```python
from build123d import *

# Parameters (mm, degrees)
SKETCH1_R           = 49.685
BOSS_EXTRUDE1_DEPTH = 5
SKETCH2_R           = 46.685
CUT_EXTRUDE1_DEPTH  = 3
SKETCH3_W           = 7
SKETCH3_H           = 5
SKETCH3_W_2         = 5
SKETCH3_H_2         = 7
BOSS_EXTRUDE2_DEPTH = 2
SKETCH4_R           = 40
BOSS_EXTRUDE3_DEPTH = 54.61
FILLET2_R           = 3
FILLET3_R           = 40


with BuildPart() as part:
    # Sketch1 → Boss-Extrude1 (new body)
    with BuildSketch(Plane.XY):
        Circle(SKETCH1_R)
    extrude(amount=BOSS_EXTRUDE1_DEPTH)

    # Sketch2 → Cut-Extrude1 (cut)
    with BuildSketch(Plane.XY.offset(5)):
        Circle(SKETCH2_R)
    extrude(amount=-CUT_EXTRUDE1_DEPTH, mode=Mode.SUBTRACT)

    # Sketch3 → Boss-Extrude2 (add)
    with BuildSketch(Plane(origin=(0, 0, 0), x_dir=(-1, 0, 0), z_dir=(0, 0, -1))):
        Polygon((-37.72768231, 37.72768231), (-67.675, 0), (-37.72768231, -37.72768231), (0, -67.675), (37.72768231, -37.72768231), (67.675, 0), (37.72768231, 37.72768231), (0, 67.675), align=None)
        with Locations((-57.675, 0)):
            Rectangle(SKETCH3_W, SKETCH3_H, mode=Mode.SUBTRACT)
        with Locations((0, 57.675)):
            Rectangle(SKETCH3_W_2, SKETCH3_H_2, mode=Mode.SUBTRACT)
        with Locations((57.675, 0)):
            Rectangle(SKETCH3_W, SKETCH3_H, mode=Mode.SUBTRACT)
        with Locations((0, -57.675)):
            Rectangle(SKETCH3_W_2, SKETCH3_H_2, mode=Mode.SUBTRACT)
    extrude(amount=BOSS_EXTRUDE2_DEPTH)

    # Sketch4 → Boss-Extrude3 (add)
    with BuildSketch(Plane(origin=(0, 0, -2), x_dir=(-1, 0, 0), z_dir=(0, 0, -1))):
        Circle(SKETCH4_R)
    extrude(amount=BOSS_EXTRUDE3_DEPTH)

    # Fillet2
    fillet2_edges = [part.edges().sort_by_distance(p)[0] for p in [
        (-67.675, 0, -1),
        (0, 67.675, -1),
        (67.675, 0, -1),
        (0, -67.675, -1),
    ]]
    fillet(fillet2_edges, radius=FILLET2_R)

    # Fillet3
    fillet3_edges = [part.edges().sort_by_distance(p)[0] for p in [
        (-37.72768231, 37.72768231, -1),
        (37.72768231, 37.72768231, -1),
        (37.72768231, -37.72768231, -1),
        (-37.72768231, -37.72768231, -1),
    ]]
    fillet(fillet3_edges, radius=FILLET3_R)


solid = part.part
```
Geometry check sheet. Reference: the model listing, model coordinates, mm. A direction names the side the tool comes from. Give positions to 0.01 mm unless a question says otherwise; leave off trailing zeros. Write each loop counter-clockwise with the first axis right and the second up, starting at its lowest first coordinate (ties: lowest second). Pieces come first, ordered by that corner, then holes. Notation, with made-up numbers: (72, 84.5) - (101, 84.5) arc R11 cw to (101, 90.5) - close; hole circle Ø5 at (84.25, 11.5). An arc over 180 degrees is marked (long way). Use a Markdown table: item, result.
Q1. Thickness scan on L1, parallel to Y at x = 0, z = 3.8 (3 decimals); L2, parallel to Z at x = -6, y = -7.5; L3, parallel to Z at x = -24.5, y = 44. Record the ranges inside material, lowest first. Write a range as [from, to].
Computed:
| item | result |
|---|---|
| L1 | y = [-49.685, -46.685], [46.685, 49.685] |
| L2 | z = [-56.61, 2] |
| L3 | z = [-2, 0] |
Q2. Go/stop test with flat-tipped pins: P1, Ø10, axis at y = 46, z = -12.5, coming from the -X side; P2, Ø2, axis at y = 26.5, z = -32.5, coming from the -X side; P3, Ø1.6, axis at x = 1, z = -0.5, coming from the -Y side; P4, Ø1, axis at y = -57.5, z = -1, coming from the -X side. Record where each tip stops, or that it passes through.
Computed:
| item | result |
|---|---|
| P1 | passes through |
| P2 | stops at x = -30.82 |
| P3 | stops at y = -66.84 |
| P4 | stops at x = -13.45 |
Q3. Set-up check for faces 1 (the face through (8.67, -39.05, -28.92)), 2 (the face through (37.587, 37.496, -1.014)), 3 (the face through (10, -49, 0)): record each of +Z, -Z, +X, -X, +Y, -Y from which the full face is reachable in a straight line by a thin tool's end or side.
Computed:
| item | result |
|---|---|
| face 1 | -Z |
| face 2 | +Z, -Z, +X, +Y |
| face 3 | +Z |
Q4. Section check D-D, the plane z = -20.5. Enter the section's corners in (x, y).
Computed:
| item | result |
|---|---|
| outline | circle Ø80 at (0, 0) |
Q5. Section check C-C, the plane y = -26.5. Enter the section's corners in (x, z), then the cut area to 3 significant figures.
Computed:
| item | result |
|---|---|
| outline | (-46.64, -2) - (-29.96, -2) - (-29.96, -56.61) - (29.96, -56.61) - (29.96, -2) - (46.64, -2) - (46.64, 0) - (42.03, 0) - (42.03, 5) - (38.43, 5) - (38.43, 2) - (-38.43, 2) - (-38.43, 5) - (-42.03, 5) - (-42.03, 0) - (-46.64, 0) - close |
| area | 3,650 mm² |
Q6. Section check A-A, the plane y = 0. Enter the section's corners in (x, z) (3 decimals), then the cut area to 3 significant figures.
Computed:
| item | result |
|---|---|
| outline | (-66.845, -2) - (-61.175, -2) - (-61.175, 0) - (-66.845, 0) - close; (-54.175, -2) - (-40, -2) - (-40, -56.61) - (40, -56.61) - (40, -2) - (54.175, -2) - (54.175, 0) - (49.685, 0) - (49.685, 5) - (46.685, 5) - (46.685, 2) - (-46.685, 2) - (-46.685, 5) - (-49.685, 5) - (-49.685, 0) - (-54.175, 0) - close; (61.175, -2) - (66.845, -2) - (66.845, 0) - (61.175, 0) - close |
| area | 4,820 mm² |
Q7. Draft check along X on faces 4 (the face through (-18.22, 53.21, -0.99)), 5 (the face through (1, 1, -56.61)), 6 (the face through (-1, 1, 2)). Enter one of: pulls with the +X half, pulls with the -X half, needs draft (parallel to the pull), parting line crosses it, or undercut.
Computed:
| item | result |
|---|---|
| face 4 | pulls with the -X half |
| face 5 | needs draft |
| face 6 | undercut |
